Autodesk Inventor part; units mm, degrees
ref_plane "YZ Plane" through (0, 0, 0) normal (1, 0, 0) x (0, 1, 0)
ref_plane "XZ Plane" through (0, 0, 0) normal (0, 1, 0) x (-1, 0, 0)
ref_plane "XY Plane" through (0, 0, 0) normal (0, 0, 1) x (1, 0, 0)
sketch "Sketch1" plane through (0, 0, 0) normal (0, 1, 0) x (-1, 0, 0)
  line L0 (0, 3.9544) -> (10, 3.9544)
  line L1 (1.5, 1.9544) -> (1.5, -36.0456)
  line L2 (1.5, -36.0456) -> (0, -36.0456)
  line L3 (0, -36.0456) -> (0, 3.9544)
  line L4 (1.5, 1.9544) -> (10, 1.9544)
  line L5 (10, 3.9544) -> (10, 1.9544)
  point P0 (0, 0)
  dimension "d0" = 10
  dimension "d1" = 2
  dimension "d2" = 40
  dimension "d21" = 1.5
revolve "Revolution1" add sketch "Sketch1" angle 360 about axis through (0, 0, -36.0456) along (0, 0, 1)
thread "Thread2"
sketch "Sketch5" plane through (0, 0, 3.9544) normal (0, 0, 1) x (1, 0, 0)
  line L0 (-3.0066, 1.7206) -> (-0.0132, 3.4641)
  line L1 (-0.0132, 3.4641) -> (2.9934, 1.7435)
  line L2 (2.9934, 1.7435) -> (3.0066, -1.7206)
  line L3 (3.0066, -1.7206) -> (0.0132, -3.4641)
  line L4 (0.0132, -3.4641) -> (-2.9934, -1.7435)
  line L5 (-2.9934, -1.7435) -> (-3.0066, 1.7206)
  circle A0 centre (0, 0) radius 18.6664
  dimension "d24" = 6
extrude "Extrusion1" cut sketch "Sketch5" against normal through all
properties part number "Fi3es60mmcsavar" material "Steel, Alloy"
Could you check a few things on this model? Use its own coordinates, in mm. A direction names the side the tool comes from. Coordinates: 2 decimals unless noted, no trailing zeros. Loops run counter-clockwise (first coordinate to the right, second up) from the corner with the lowest first, then second, coordinate; pieces in that order, holes last.
1) Imagine slicing it at B-B (x = 1). List the corners of the cut face in (y, z) for me.
Reported:
outline: (-2.89, 1.95) - (-1.12, 1.95) - (-1.12, -36.05) - (1.12, -36.05) - (1.12, 1.95) - (2.88, 1.95) - (2.88, 3.95) - (-2.89, 3.95) - close
2) Imagine slicing it at A-A (y = 0). List the corners of the cut face in (x, z) for me.
Reported:
outline: (-3, 1.95) - (-1.5, 1.95) - (-1.5, -36.05) - (1.5, -36.05) - (1.5, 1.95) - (3, 1.95) - (3, 3.95) - (-3, 3.95) - close
3) Will these pins go through, and if not, where does the flat tip stop? pin 1 Ø2 at (x, z) = (1.5, -30.5) entering from -Y; pin 2 Ø4 at (y, z) = (-0.5, -11.5) entering from +X.
Reported:
pin 1: stops at y = -1.41
pin 2: stops at x = 1.5
4) Which directions (+Z, -Z, +X, -X, +Y, -Y) give clear straight access to the entire face, cutting with the end or side of a thin tool? Please do faces 1 (the face through (-1.5, 2.6, 3)), 2 (the face through (0.7, 1.5, 1.954)).
Reported:
face 1: +Z, -Z, -X, +Y
face 2: -Z
5) Imagine slicing it at C-C (z = -20). List the corners of the cut face in (x, y) for me, and give its area (3 significant figures).
Reported:
outline: circle Ø3 at (0, 0)
area: 7.07 mm2
6) Please list where these lines run through material, in increasing order: line 1 along Z through (x, y) = (1.75, 0.25); line 2 along Y through (x, z) = (0, -33); line 3 along Y through (x, z) = (1.25, -17).
Reported:
line 1: z = 1.95 to 3.95
line 2: y = -1.5 to 1.5
line 3: y = -0.83 to 0.83
